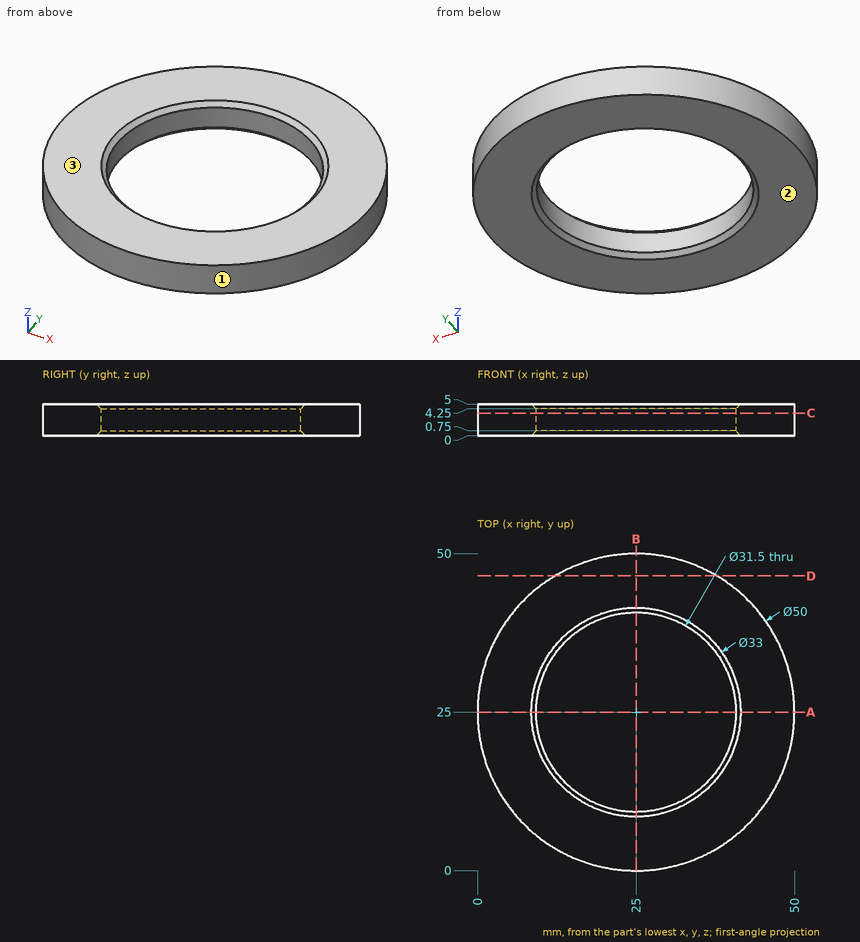
Design review of the part shown in the three views and the two pictorial views. Dimensions are in mm from the part's minimum x, y and z. Give positions to 0.01 mm unless a question says otherwise; leave off trailing zeros. Loops run counter-clockwise (first coordinate to the right, second up) from the corner with the lowest first, then second, coordinate; pieces in that order, holes last. Notation, with made-up numbers: M 67,5.25 L 95,5.25 A20 ccw 95,22.25 Z; hole C 44.25,-14 d3. An arc over 180 degrees is marked long. Answer as a JSON object with one key per item and string values. Group by question number.
Q1. Add section C-C on z = 3.55. Give the boundary of the cut face in (x, y), and give its area (3 significant figures).
Q2. Add section D-D on y = 46.5. Give the boundary of the cut face in (x, z).
Q3. Mouldability with a two-part tool opening along Z and no side actions: class the marked faces 1, 2 and 3 as +Z half, -Z half, draft (parallel to the pull), parting line (faces both ways), or undercut.
Q4. For probe 1 along Y at (x, z) = (25, 2); probe 2 along X at (y, z) = (11, 0.3); probe 3 along X at (y, z) = (38.5, 1.65), list the stretches that pass through material, from the lowest coordinate up. Write a range as [from, to].
Q5. Add section A-A on y = 25. Give the boundary of the cut face in (x, z).
Q6. Insertion check: P1, Ø1.5, axis at y = 27, z = 2.5, coming from the -X side. The pin has a flat end and moves straight along its axis. Give the tip position at first contact, or say it passes through.
Checked values:
{
 "1": {"outline": "C 25,25 d50; hole C 25,25 d31.5", "area": "1,180 mm²"},
 "2": {"outline": "M 12.24,0 L 37.76,0 L 37.76,5 L 12.24,5 Z"},
 "3": {"face 1": "draft", "face 2": "-Z half", "face 3": "+Z half"},
 "4": {"probe 1": "[0, 9.25], [40.75, 50]", "probe 2": "[4.29, 16.85], [33.15, 45.71]", "probe 3": "[3.96, 16.89], [33.11, 46.04]"},
 "5": {"outline": "M 0,0 L 8.5,0 L 9.25,0.75 L 9.25,4.25 L 8.5,5 L 0,5 Z; M 40.75,0.75 L 41.5,0 L 50,0 L 50,5 L 41.5,5 L 40.75,4.25 Z"},
 "6": {"P1": "x = 0.03"}
}
